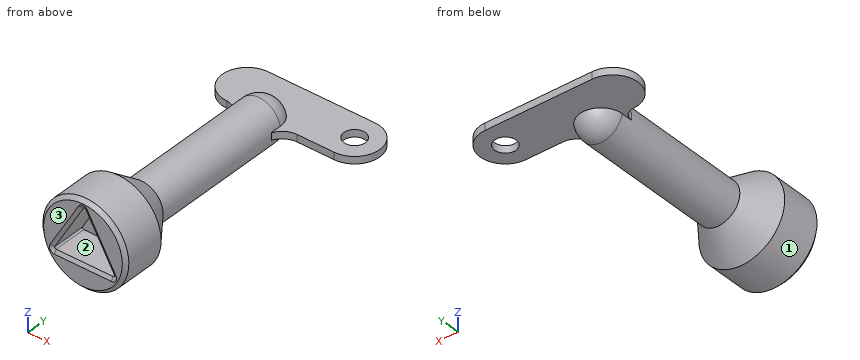
```python
from build123d import *

# Parameters (mm, degrees)
SKETCH_1_R          = 6
EXTRUDE_1_DEPTH     = 6
SKETCH_2_R          = 3
SKETCH_1_2_R        = 6
SKETCH_2_2_R        = 3
EXTRUDE_2_DEPTH     = 20
EXTRUDE_4_DEPTH     = 0.5
SKETCH_8_R          = 1.5
CUT_EXTRUDE_1_DEPTH = 35.630189161
CUT_EXTRUDE_2_DEPTH = 5
CHAMFER_1_SIZE      = 0.5
CHAMFER_1_SIZE2     = 0.288675135
CHAMFER_2_SIZE      = 0.5


with BuildPart() as part:
    # 草图1 → 凸台-拉伸1 (new body)
    with BuildSketch(Plane(origin=(0, 0, 0), x_dir=(1, 0, 0), z_dir=(0, 1, 0))):
        with Locations(Location((0, 0, 0), (0, 0, 270))):
            Circle(SKETCH_1_R)
    extrude(amount=-EXTRUDE_1_DEPTH)

    # 草图2 → 放样1 section 0
    with BuildSketch(Plane(origin=(0, 4, 0), x_dir=(1, 0, 0), z_dir=(0, 1, 0))):
        Circle(SKETCH_2_R)
    # 草图1<2> → 放样1 section 1
    with BuildSketch(Plane(origin=(0, 0, 0), x_dir=(1, 0, 0), z_dir=(0, 1, 0))):
        Circle(SKETCH_1_2_R)
    loft()

    # 草图2<2> → 凸台-拉伸2 (add)
    with BuildSketch(Plane(origin=(0, 4, 0), x_dir=(1, 0, 0), z_dir=(0, 1, 0))):
        with Locations(Location((0, 0, 0), (0, 0, 270))):
            Circle(SKETCH_2_2_R)
    extrude(amount=EXTRUDE_2_DEPTH)

    # 草图7 → 旋转2 (revolve)
    with BuildSketch(Plane.XY, mode=Mode.PRIVATE) as revolve_2_sk:
        with BuildLine():
            Line((-3, 24), (0, 24))
            Line((0, 24), (0, 27))
            ThreePointArc((0, 27), (-2.121320344, 26.121320344), (-3, 24))
        make_face()
    revolve(revolve_2_sk.sketch.rotate(Axis((0, 0, 0), (0, 1, 0)), 90), axis=Axis((0, 0, 0), (0, 1, 0)))

    # 草图5 → 凸台-拉伸4 (add, symmetric)
    with BuildSketch(Plane.XY):
        with BuildLine():
            Line((-3, 22.5), (3, 22.5))
            ThreePointArc((3, 22.5), (3.921981454, 23.591650066), (5.291287847, 24))
            Line((5.291287847, 24), (10.5, 24))
            ThreePointArc((10.5, 24), (14, 27.5), (10.5, 31))
            Line((10.5, 31), (-4.5, 31))
            ThreePointArc((-4.5, 31), (-8, 27.5), (-4.5, 24))
            ThreePointArc((-4.5, 24), (-3.439339828, 23.560660172), (-3, 22.5))
        make_face()
    extrude(amount=EXTRUDE_4_DEPTH, both=True)

    # 草图8 → 切除-拉伸1 (cut, through all)
    with BuildSketch(Plane.XY.offset(0.5)):
        with Locations((10.5, 27.5)):
            Circle(SKETCH_8_R)
    extrude(amount=-CUT_EXTRUDE_1_DEPTH, mode=Mode.SUBTRACT)

    # 草图9 → 切除-拉伸2 (cut)
    with BuildSketch(Plane.XZ.offset(6)):
        with BuildLine():
            Line((-0.173205081, 4.7), (-4.156921938, -2.2))
            ThreePointArc((-4.156921938, -2.2), (-4.156921938, -2.4), (-3.983716857, -2.5))
            Line((-3.983716857, -2.5), (3.983716857, -2.5))
            ThreePointArc((3.983716857, -2.5), (4.156921938, -2.4), (4.156921938, -2.2))
            Line((4.156921938, -2.2), (0.173205081, 4.7))
            ThreePointArc((0.173205081, 4.7), (0, 4.8), (-0.173205081, 4.7))
        make_face()
    extrude(amount=-CUT_EXTRUDE_2_DEPTH, mode=Mode.SUBTRACT)

    # 倒角1
    chamfer_1_edges = [part.edges().sort_by_distance(p)[0] for p in [
        (4.156921938, -6, -2.4),
        (2.165063509, -6, 1.25),
        (0, -6, 4.8),
        (-2.165063509, -6, 1.25),
        (-4.156921938, -6, -2.4),
        (0, -6, -2.5),
    ]]
    chamfer_1_side = [part.faces().sort_by_distance(p)[0] for p in [
        (0, -6, -5.830294373),
    ]]
    chamfer(chamfer_1_edges, length=CHAMFER_1_SIZE, length2=CHAMFER_1_SIZE2, reference=chamfer_1_side[0])

    # 倒角2
    chamfer_2_edges = [part.edges().sort_by_distance(p)[0] for p in [
        (0, -6, -6),
    ]]
    chamfer(chamfer_2_edges, length=CHAMFER_2_SIZE)


solid = part.part
```
CAD build for the part. Positions are in the model's coordinates, mm. Face numbers are marked on the shaded views. Give positions to 0.01 mm unless a question says otherwise; leave off trailing zeros. Order: outer loops, then holes, each group sorted by start corner. A loop starts at its lowest first (then second) coordinate and runs counter-clockwise, first axis right, second up.
(1) Mould opens along X. For the marked faces 1, 2 and 3 say: released by +X, released by -X, zero draft, split by the parting line, or undercut.
(2) Saw through at D-D, the plane x = 6.5. Give the cut face in (y, z), then the cut area to 3 significant figures.
(3) Saw through at C-C, the plane y = 5. Give the cut face in (x, z), then the cut area to 3 significant figures.
(4) Saw through at A-A, the plane y = 27.5. Give the cut face in (x, z).
(5) Drill centre lines: L1, parallel to Y at x = 10.5, z = 0.3; L2, parallel to Z at x = 4.75, y = 25.5; L3, parallel to Z at x = 3.5, y = -2. Where is each one in solid material? Low to high.
(6) Saw through at B-B, the plane x = 10. Give the cut face in (y, z).
(7) Flat gauge pins, fed straight in: pin 1 (1 mm diameter, centred on y = 5, z = 0, fed in from -X); pin 2 (9.5 mm diameter, centred on x = 0.5, y = 28.5, fed in from +Z); pin 3 (0.5 mm diameter, centred on x = 8, z = 0, fed in from -Y); pin 4 (5 mm diameter, centred on x = -4.5, z = -4, fed in from -Y). Where does each tip first touch, or does it go through?
Results found:
1. face 1: split by the parting line
1. face 2: undercut
1. face 3: zero draft
2. outline: (24, -0.5) - (31, -0.5) - (31, 0.5) - (24, 0.5) - close
2. area: 7.00 mm2
3. outline: circle Ø6 at (0, 0)
3. area: 28.3 mm2
4. outline: (-8, -0.5) - (9, -0.5) - (9, 0.5) - (-8, 0.5) - close; (12, -0.5) - (14, -0.5) - (14, 0.5) - (12, 0.5) - close
5. L1: y = 24 to 26, 29 to 31
5. L2: z = -0.5 to 0.5
5. L3: z = -4.87 to -2.5, -1.06 to 4.87
6. outline: (24, -0.5) - (26.09, -0.5) - (26.09, 0.5) - (24, 0.5) - close; (28.91, -0.5) - (31, -0.5) - (31, 0.5) - (28.91, 0.5) - close
7. pin 1: stops at x = -3
7. pin 2: stops at z = 3
7. pin 3: stops at y = 24
7. pin 4: stops at y = -6
